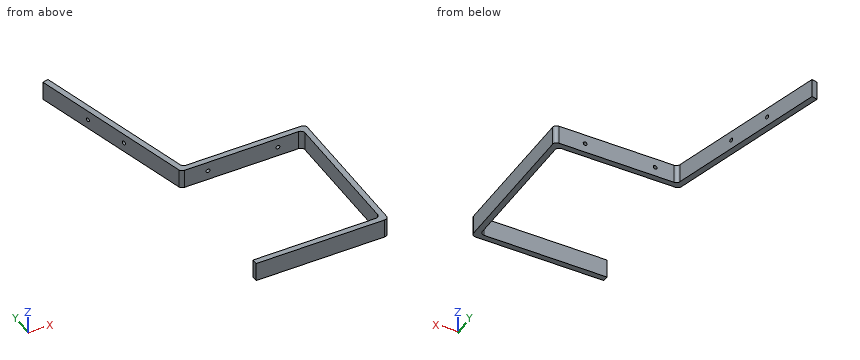
from build123d import *

# Parameters (mm, degrees)
BOSS_EXTRUDE1_DEPTH = 25
SKETCH3_R           = 5
CUT_EXTRUDE1_DEPTH  = 20
SKETCH2_R           = 5
CUT_EXTRUDE2_DEPTH  = 20


with BuildPart() as part:
    # Sketch1 → Boss-Extrude1 (new body, symmetric)
    with BuildSketch(Plane.XY):
        with BuildLine():
            Line((-388.398049097, -14.110780444), (-502.733667869, 412.59555793))
            Line((-502.733667869, 412.59555793), (-517.733667869, 408.576320044))
            Line((-517.733667869, 408.576320044), (-400.48638755, -29.110107171))
            ThreePointArc((-400.48638755, -29.110107171), (-396.65053803, -34.851466611), (-390.112163796, -37.0710639))
            Line((-390.112163796, -37.0710639), (-89.247234395, -37.0710639))
            ThreePointArc((-89.247234395, -37.0710639), (-81.652907565, -40.21673707), (-78.507234395, -47.8110639))
            Line((-78.507234395, -47.8110639), (-78.507234395, -396.3310639))
            ThreePointArc((-78.507234395, -396.3310639), (-81.652907565, -403.92539073), (-89.247234395, -407.0710639))
            Line((-89.247234395, -407.0710639), (-412.734449588, -407.0710639))
            Line((-412.734449588, -407.0710639), (-412.734449588, -422.0710639))
            Line((-412.734449588, -422.0710639), (-74.247234395, -422.0710639))
            ThreePointArc((-74.247234395, -422.0710639), (-66.652907565, -418.92539073), (-63.507234395, -411.3310639))
            Line((-63.507234395, -411.3310639), (-63.507234395, -32.8110639))
            ThreePointArc((-63.507234395, -32.8110639), (-66.652907565, -25.21673707), (-74.247234395, -22.0710639))
            Line((-74.247234395, -22.0710639), (-378.024005722, -22.0710639))
            ThreePointArc((-378.024005722, -22.0710639), (-384.56210347, -19.851678775), (-388.398049097, -14.110780444))
        make_face()
    extrude(amount=BOSS_EXTRUDE1_DEPTH, both=True)

    # Sketch3 → Cut-Extrude1 (cut)
    with BuildSketch(Plane(origin=(0, -22.0710639, 0), x_dir=(1, 0, 0), z_dir=(0, 1, 0))):
        with Locations((-327.977212353, 0)):
            Circle(SKETCH3_R)
        with Locations((-143.507234395, 0)):
            Circle(SKETCH3_R)
    extrude(amount=-CUT_EXTRUDE1_DEPTH, mode=Mode.SUBTRACT)

    # Sketch2 → Cut-Extrude2 (cut)
    with BuildSketch(Plane(origin=(-365.908008308, -98.04475533, 0), x_dir=(0, 0, -1), z_dir=(0.965925826, 0.258819045, 0))):
        with Locations((0, 378.653753076)):
            Circle(SKETCH2_R)
        with Locations((0, 258.653753076)):
            Circle(SKETCH2_R)
    extrude(amount=-CUT_EXTRUDE2_DEPTH, mode=Mode.SUBTRACT)


solid = part.part
Verification items for the finished model (mm, model axes). Coordinates: 2 decimals unless noted, no trailing zeros. Order: outer loops, then holes, each group sorted by start corner. A loop starts at its lowest first (then second) coordinate and runs counter-clockwise, first axis right, second up.
Item 1: Depth check by flat-ended pin: pin 1 (11.5 mm diameter, centred on x = -327.98, z = 0, fed in from +Y); pin 2 (6 mm diameter, centred on y = 288, z = -15.5, fed in from +X); pin 3 (1 mm diameter, centred on y = 261.5, z = 15.5, fed in from -X). Enter the tip coordinate at first touch or a pass-through.
Filled in:
pin 1: stops at y = -22.07
pin 2: stops at x = -468.54
pin 3: stops at x = -478.47
Item 2: Section check D-D, the plane y = 167.5. Enter the section's corners in (x, z).
Filled in:
outline: (-453.15, -25) - (-437.06, -25) - (-437.06, 25) - (-453.15, 25) - close
Item 3: Section check A-A, the plane x = -269.5. Enter the section's corners in (y, z).
Filled in:
outline: (-422.07, -25) - (-407.07, -25) - (-407.07, 25) - (-422.07, 25) - close; (-37.07, -25) - (-22.07, -25) - (-22.07, 25) - (-37.07, 25) - close
Item 4: Material ranges on L1, parallel to Y at x = -254, z = 6.5; L2, parallel to X at y = -26, z = 0; L3, parallel to X at y = -33, z = 0, recorded low to high.
Filled in:
L1: y = -422.07 to -407.07, -37.07 to -22.07
L2: x = -401.32 to -332.98, -322.98 to -148.51, -138.51 to -65.94
L3: x = -398.53 to -332.98, -322.98 to -148.51, -138.51 to -63.51
Item 5: Section check C-C, the plane y = -259. Enter the section's corners in (x, z).
Filled in:
outline: (-78.51, -25) - (-63.51, -25) - (-63.51, 25) - (-78.51, 25) - close
Item 6: Section check B-B, the plane z = 17.5. Enter the section's corners in (x, y), then the cut area to 3 significant figures.
Filled in:
outline: (-517.73, 408.58) - (-400.49, -29.11) arc R10.74 ccw to (-390.11, -37.07) - (-89.25, -37.07) arc R10.74 cw to (-78.51, -47.81) - (-78.51, -396.33) arc R10.74 cw to (-89.25, -407.07) - (-412.73, -407.07) - (-412.73, -422.07) - (-74.25, -422.07) arc R10.74 ccw to (-63.51, -411.33) - (-63.51, -32.81) arc R10.74 ccw to (-74.25, -22.07) - (-378.02, -22.07) arc R10.74 cw to (-388.4, -14.11) - (-502.73, 412.6) - close
area: 22,800 mm2
